Read the model definition and answer for the solid it produces. Units are mm, in the model's axes. Face numbers are marked on the shaded views. A direction names the side the tool comes from. Coordinates: 2 decimals unless noted, no trailing zeros. Write each loop counter-clockwise with the first axis right and the second up, starting at its lowest first coordinate (ties: lowest second). Pieces come first, ordered by that corner, then holes.
1) The part is cut by section B-B (y = 99). Determine the outline of the cut face in (x, z), then the cut area to 3 significant figures.
2) The part is cut by section D-D (z = -19.75). Determine the outline of the cut face in (x, y), then the cut area to 3 significant figures.
3) Determine the mould class of the marked faces 1, 2 and 3 for opening direction Z: +Z half, -Z half, draft (parallel to the pull), parting line (faces both ways), or undercut.
4) Which of the six approach directions +Z, -Z, +X, -X, +Y, -Y give full straight-line access (tool end or side, diameter ignored) to the marked faces 4, 5 and 6?
5) Find the intervals of material crossed by line 1 (Y direction, x = -2, z = -5.75); line 2 (Y direction, x = -3.75, z = -17); line 3 (X direction, y = 115.5, z = -3), in increasing order.
6) Each of these flat-tipped pins is pushed along its axis until it touches: pin 1 Ø5.5 at (y, z) = (105, -5.5) entering from +X; pin 2 Ø1.8 at (x, z) = (3, -18.5) entering from +Y; pin 3 Ø2 at (y, z) = (92.5, -7) entering from +X. Where does it stop, or does it pass through?
7) The part is cut by section A-A (x = -2.25). Determine the outline of the cut face in (y, z), then the cut area to 3 significant figures.
from build123d import *

# Parameters (mm, degrees)
BOSS_EXTRUDE1_DEPTH = 100
BOSS_EXTRUDE2_DEPTH = 10
BOSS_EXTRUDE2_DRAFT = 45
SKETCH3_R           = 34.5
BOSS_EXTRUDE3_DEPTH = 10
SKETCH4_R           = 31
BOSS_EXTRUDE4_DEPTH = 30
SKETCH5_R           = 2
CUT_EXTRUDE1_DEPTH  = 5
CIRPATTERN1_COUNT   = 12
BOSS_EXTRUDE5_DEPTH = 100
SKETCH7_R           = 31
BOSS_EXTRUDE6_DEPTH = 10
SKETCH8_R           = 30
BOSS_EXTRUDE7_DEPTH = 11
SKETCH10_R          = 42.5
BOSS_EXTRUDE8_DEPTH = 10.5
BOSS_EXTRUDE9_DEPTH = 55
SKETCH12_R          = 15
CUT_EXTRUDE2_DEPTH  = 20
SKETCH13_R          = 15
CUT_EXTRUDE3_DEPTH  = 20
L_EK1_SCALE         = 0.2


with BuildPart() as part:
    # Sketch1 → Boss-Extrude1 (new body)
    with BuildSketch(Plane(origin=(0, 0, 0), x_dir=(1, 0, 0), z_dir=(0, 1, 0))):
        with BuildLine():
            Line((-37.5, 45), (37.5, 45))
            ThreePointArc((37.5, 45), (45.880962103, 0), (37.5, -45))
            Line((37.5, -45), (-37.5, -45))
            ThreePointArc((-37.5, -45), (-45.880962103, 0), (-37.5, 45))
        make_face()
    extrude(amount=BOSS_EXTRUDE1_DEPTH)


with BuildPart() as boss_extrude2_tool:
    # Sketch2 → Boss-Extrude2 (with draft: the straight prism first)
    with BuildSketch(Plane(origin=(0, 100, 0), x_dir=(1, 0, 0), z_dir=(0, 1, 0))):
        with BuildLine():
            Line((-37.5, -45), (37.5, -45))
            ThreePointArc((37.5, -45), (45.880962103, 0), (37.5, 45))
            Line((37.5, 45), (-37.5, 45))
            ThreePointArc((-37.5, 45), (-45.880962103, 0), (-37.5, -45))
        make_face()
    extrude(amount=BOSS_EXTRUDE2_DEPTH)
    # Boss-Extrude2: the draft: its side faces are tilted about the plane it starts from
    boss_extrude2_sides = [boss_extrude2_tool.faces().sort_by_distance(p)[0] for p in [
        (0, 105, -45),
        (-45.880962103, 105, 0),
        (0, 105, 45),
        (45.880962103, 105, 0),
    ]]
    draft(boss_extrude2_sides, Plane(origin=(0, 100, 0), x_dir=(1, 0, 0), z_dir=(0, 1, 0)), BOSS_EXTRUDE2_DRAFT)


with BuildPart() as part_1:
    add(part.part)

    # Boss-Extrude2: add boss_extrude2_tool
    add(boss_extrude2_tool.part)

    # Sketch3 → Boss-Extrude3 (add)
    with BuildSketch(Plane(origin=(0, 110, 0), x_dir=(1, 0, 0), z_dir=(0, 1, 0))):
        with Locations(Location((0, 0, 0), (0, 0, 270))):
            Circle(SKETCH3_R)
    extrude(amount=BOSS_EXTRUDE3_DEPTH)

    # Sketch4 → Boss-Extrude4 (add)
    with BuildSketch(Plane(origin=(0, 120, 0), x_dir=(1, 0, 0), z_dir=(0, 1, 0))):
        with Locations(Location((0, 0, 0), (0, 0, 270))):
            Circle(SKETCH4_R)
    extrude(amount=BOSS_EXTRUDE4_DEPTH)

    # Sketch5 → Cut-Extrude1 (cut)
    with BuildSketch(Plane(origin=(0, 150, 0), x_dir=(1, 0, 0), z_dir=(0, 1, 0))):
        with Locations(Location((27, 0, 0), (0, 0, 270))):
            Circle(SKETCH5_R)
    cut_extrude1 = extrude(amount=-CUT_EXTRUDE1_DEPTH, mode=Mode.SUBTRACT)

    # CirPattern1: Cut-Extrude1 ×12 about axis
    cirpattern1_axis = Axis((-0.112852665, 0, 0), (0, 1, 0))
    for i in range(1, CIRPATTERN1_COUNT):
        add(cut_extrude1.rotate(cirpattern1_axis, i * 360 / CIRPATTERN1_COUNT), mode=Mode.SUBTRACT)

    # Sketch6 → Boss-Extrude5 (add)
    with BuildSketch(Plane(origin=(0, 150, 0), x_dir=(1, 0, 0), z_dir=(0, 1, 0))):
        with BuildLine():
            Line((-16, -17), (-16, 17))
            ThreePointArc((-16, 17), (0, 23.900331129), (16, 17))
            Line((16, 17), (16, -17))
            ThreePointArc((16, -17), (0, -23.900331129), (-16, -17))
        make_face()
    extrude(amount=BOSS_EXTRUDE5_DEPTH)

    # Sketch7 → Boss-Extrude6 (add)
    with BuildSketch(Plane(origin=(0, 250, 0), x_dir=(1, 0, 0), z_dir=(0, 1, 0))):
        with Locations(Location((0, 0, 0), (0, 0, 270))):
            Circle(SKETCH7_R)
    extrude(amount=BOSS_EXTRUDE6_DEPTH)

    # Sketch8 → Boss-Extrude7 (add)
    with BuildSketch(Plane(origin=(0, 260, 0), x_dir=(1, 0, 0), z_dir=(0, 1, 0))):
        with Locations(Location((0, 0, 0), (0, 0, 270))):
            Circle(SKETCH8_R)
    extrude(amount=BOSS_EXTRUDE7_DEPTH)

    # Sketch10 → Boss-Extrude8 (add, symmetric)
    with BuildSketch(Plane(origin=(37.5, 0, 0), x_dir=(0, 0, -1), z_dir=(1, 0, 0))):
        with Locations(Location((45, 50, 0), (0, 0, 90))):
            Circle(SKETCH10_R)
    extrude(amount=BOSS_EXTRUDE8_DEPTH, both=True)

    # Sketch11 → Boss-Extrude9 (add)
    with BuildSketch(Plane.ZY.offset(-27)):
        with BuildLine():
            Line((-45, 30), (-75, 30))
            ThreePointArc((-75, 30), (-82.639320225, 50), (-75, 70))
            Line((-75, 70), (-45, 70))
            Line((-45, 70), (-45, 30))
        make_face()
    extrude(amount=BOSS_EXTRUDE9_DEPTH)

    # Sketch12 → Cut-Extrude2 (cut)
    with BuildSketch(Plane(origin=(0, 271, 0), x_dir=(1, 0, 0), z_dir=(0, 1, 0))):
        with Locations(Location((0, 0, 0), (0, 0, 270))):
            Circle(SKETCH12_R)
    extrude(amount=-CUT_EXTRUDE2_DEPTH, mode=Mode.SUBTRACT)

    # Sketch13 → Cut-Extrude3 (cut)
    with BuildSketch(Plane(origin=(48, 0, 0), x_dir=(0, 0, -1), z_dir=(1, 0, 0))):
        with Locations((45, 50)):
            Circle(SKETCH13_R)
    extrude(amount=-CUT_EXTRUDE3_DEPTH, mode=Mode.SUBTRACT)


with BuildPart() as part_2:
    # Ölçek1: scaled about (1.834934624, 84.278783532, -6.572274509)
    add(part_1.part.scale(L_EK1_SCALE).moved(Location((1.467947699, 67.423026826, -5.257819607))))


solid = part_2.part
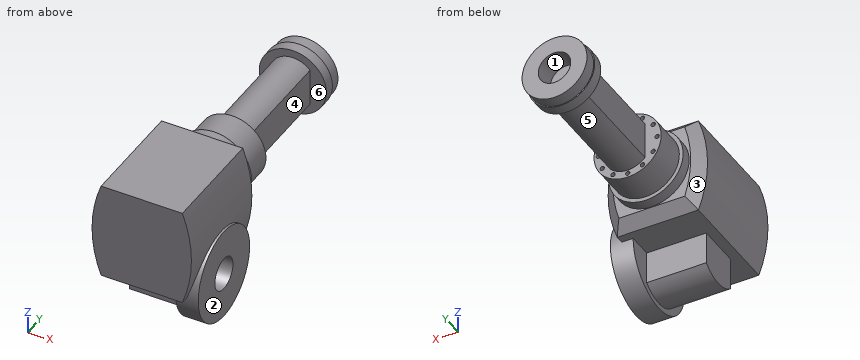
Reported:
1. outline: (-1.73, -8.66) arc R4.4 ccw to (4.67, -8.66) - (4.67, -1.86) arc R4.4 ccw to (-1.73, -1.86) - close
1. area: 55.7 mm2
2. outline: (-4.13, 73.42) - (6.87, 73.42) - (6.87, 70.94) - (11.07, 70.94) - (11.07, 83.91) - (6.87, 83.91) - (6.87, 81.42) - (-4.13, 81.42) - close
2. area: 142 mm2
3. face 1: undercut
3. face 2: draft
3. face 3: parting line
4. face 4: +Z, -Z, +X
4. face 5: -Z
4. face 6: none
5. line 1: y = 67.42 to 97.42, 117.42 to 121.62
5. line 2: y = 73.42 to 81.42
5. line 3: x = -1.73 to 4.67
6. pin 1: stops at x = 4.67
6. pin 2: stops at y = 81.42
6. pin 3: stops at x = 7.62
7. outline: (67.42, -14.26) - (73.42, -14.26) - (73.42, -20.26) arc R6 ccw to (81.42, -20.26) - (81.42, -14.26) - (87.42, -14.26) - (89.42, -12.26) - (89.42, -11.07) - (91.42, -11.07) - (91.42, -10.22) - (97.42, -10.22) - (97.42, -0.3) - (91.42, -0.3) - (91.42, 0.55) - (89.42, 0.55) - (89.42, 1.74) - (87.42, 3.74) - (67.42, 3.74) - close; (117.42, -10.22) - (119.42, -10.22) - (119.42, -9.97) - (121.62, -9.97) - (121.62, -0.55) - (119.42, -0.55) - (119.42, -0.3) - (117.42, -0.3) - close
7. area: 572 mm2
